Build history of the part. All positions in model axes, mm. A direction names the side the tool comes from. Coordinates: 2 decimals unless noted, no trailing zeros. Order: outer loops, then holes, each group sorted by start corner. A loop starts at its lowest first (then second) coordinate and runs counter-clockwise, first axis right, second up. Notation, with made-up numbers: (48, 81.5) -> (105, 81.5) arc R21 cw to (105, 93.5) -> close; hole circle Ø10 at (87, 52.5). An arc over 180 degrees is marked (long way). Write each question's results on one line, items separated by ' | '.
from build123d import *

# Parameters (mm, degrees)
F1_DEPTH = 40
F2_R     = 12.6
F3_T     = -4.129
F5_DEPTH = 14
F6_DEPTH = 20.001
F7_R     = 4.4681980282
F8_DEPTH = 12


with BuildPart() as f1:
    # F0 (on Top) → F1 (new body)
    with BuildSketch(Plane.XY):
        Polygon((-75.5, -10), (75.5, -10), (71.5217526524, 10), (-71.5217526524, 10), align=None)
    extrude(amount=F1_DEPTH)

    # F2
    f2_edges = [f1.edges().sort_by_distance(p)[0] for p in [
        (-71.521753, 10, 20),
        (0, 10, 40),
        (0, 10, 0),
        (71.521753, 10, 20),
        (-73.510876, 0, 40),
        (-73.510876, 0, 0),
        (73.510876, 0, 40),
        (73.510876, 0, 0),
    ]]
    fillet(f2_edges, radius=F2_R)

    # F3
    f3_openings = [f1.faces().sort_by_distance(p)[0] for p in [
        (0, -10, 20),
    ]]
    offset(amount=F3_T, openings=f3_openings)

    # F4 (on face) → F5 (join)
    with BuildSketch(Plane.XZ.offset(10)):
        with BuildLine():
            ThreePointArc((-71.2901081078, 22.15), (-69.7698285282, 21.5202795796), (-69.1401081078, 20))
            ThreePointArc((-69.1401081078, 20), (-69.7698285282, 18.4797204204), (-71.2901081078, 17.85))
            Line((-71.2901081078, 17.85), (-71.2901081078, 12.6))
            ThreePointArc((-71.2901081078, 12.6), (-63.8901081078, 20), (-71.2901081078, 27.4))
            Line((-71.2901081078, 27.4), (-71.2901081078, 22.15))
        make_face()
        with BuildLine():
            Line((71.2901081078, 22.15), (71.2901081078, 27.4))
            ThreePointArc((71.2901081078, 27.4), (63.8901081078, 20), (71.2901081078, 12.6))
            Line((71.2901081078, 12.6), (71.2901081078, 17.85))
            ThreePointArc((71.2901081078, 17.85), (69.1401081078, 20), (71.2901081078, 22.15))
        make_face()
    extrude(amount=-F5_DEPTH)

    # F4 (on face) → F6 (cut, through all)
    with BuildSketch(Plane.XZ.offset(10)):
        with BuildLine():
            ThreePointArc((-71.2901081078, 17.85), (-69.7698285282, 18.4797204204), (-69.1401081078, 20))
            ThreePointArc((-69.1401081078, 20), (-69.7698285282, 21.5202795796), (-71.2901081078, 22.15))
            Line((-71.2901081078, 22.15), (-71.2901081078, 17.85))
        make_face()
        with BuildLine():
            Line((-71.2901081078, 17.85), (-71.2901081078, 22.15))
            ThreePointArc((-71.2901081078, 22.15), (-73.4401081078, 20), (-71.2901081078, 17.85))
        make_face()
        with BuildLine():
            ThreePointArc((73.4401081078, 20), (72.8103876873, 21.5202795796), (71.2901081078, 22.15))
            Line((71.2901081078, 22.15), (71.2901081078, 17.85))
            ThreePointArc((71.2901081078, 17.85), (72.8103876873, 18.4797204204), (73.4401081078, 20))
        make_face()
        with BuildLine():
            Line((71.2901081078, 17.85), (71.2901081078, 22.15))
            ThreePointArc((71.2901081078, 22.15), (69.1401081078, 20), (71.2901081078, 17.85))
        make_face()
    extrude(amount=-F6_DEPTH, mode=Mode.SUBTRACT)

    # F7 (on face) → F8 (cut)
    with BuildSketch(Plane(origin=(0, 10, 0), x_dir=(-1, 0, 0), z_dir=(0, 1, 0))):
        with Locations((71.2666511536, 20.0136322528)):
            Circle(F7_R)
        with Locations((-71.2666511536, 20.0136322528)):
            Circle(F7_R)
    extrude(amount=-F8_DEPTH, mode=Mode.SUBTRACT)


solid = f1.part
Item 1: Tool access for faces 1 (the flat face through (-68.7, -2, 20.1)), 2 (the flat face through (65, 4, 20)), 3 (the flat face through (-1, -6, 40)), 4 (the cylindrical face through (-0.86, 3.46, 33.32)), 5 (the flat face through (74.533, -5.14, 19.896)): list every direction of +Z, -Z, +X, -X, +Y, -Y with a clear straight run to the whole face (end or side of a thin tool).
Answer:
face 1: +Y | face 2: none | face 3: +Z, +X, -X, +Y, -Y | face 4: -Y | face 5: +Z, -Z, +X, +Y
Item 2: Pin check, flat tips, straight feed: pin 1 (6 mm diameter, centred on y = 5.5, z = 16.5, fed in from -X); pin 2 (2 mm diameter, centred on x = 65, z = 22, fed in from +Y); pin 3 (0.8 mm diameter, centred on x = -65, z = 22, fed in from +Y). Stop position of each tip, or through.
Answer:
pin 1: stops at x = -72.66 | pin 2: stops at y = 9.68 | pin 3: stops at y = 9.53
Item 3: Slice it at B-B, the plane z = 8. List the corners of the cut face in (x, y).
Answer:
outline: (-74.61, -10) -> (-69.91, -10) -> (-68.16, -1.21) arc R7.11 cw to (-61.18, 4.51) -> (61.18, 4.51) arc R7.11 cw to (68.16, -1.21) -> (69.91, -10) -> (74.61, -10) -> (72.69, -0.31) arc R11.73 ccw to (61.18, 9.13) -> (-61.18, 9.13) arc R11.73 ccw to (-72.69, -0.31) -> close
Item 4: Slice it at A-A, the plane x = 7. List the corners of the cut face in (y, z), and give its area (3 significant figures).
Answer:
outline: (-10, 0) -> (-2.6, 0) arc R12.6 ccw to (10, 12.6) -> (10, 27.4) arc R12.6 ccw to (-2.6, 40) -> (-10, 40) -> (-10, 35.87) -> (-2.6, 35.87) arc R8.47 cw to (5.87, 27.4) -> (5.87, 12.6) arc R8.47 cw to (-2.6, 4.13) -> (-10, 4.13) -> close | area: 259 mm^2
Item 5: Pull direction X, two halves, no side cores. Call faces 6 (the cylindrical face through (-65.76, 9.14, 20.1)), 7 (the cylindrical face through (-63.89, -3.1, 19.84)), 8 (the cylindrical face through (-0.86, 6.41, 36.21)): released by +X, released by -X, zero draft, split by the parting line, or undercut.
Answer:
face 6: released by -X | face 7: undercut | face 8: zero draft
Item 6: Slice it at C-C, the plane y = -7.25. State how many separate pieces and enclosed holes the cut face has, and give its area (3 significant figures).
Answer:
separate pieces: 1 | enclosed holes: 3 | area: 1,560 mm^2
Item 7: Drill centre lines: line 1 (Z direction, x = 1, y = -2.25); line 2 (X direction, y = -6.25, z = 20); line 3 (X direction, y = -6.75, z = 20). Where is each one in solid material? Low to high. Write a range as from..to.
Answer:
line 1: z = 0..4.14, 35.86..40 | line 2: x = -74.75..-73.44, -69.14..-63.89, 63.89..69.14, 73.44..74.75 | line 3: x = -74.85..-73.44, -69.14..-63.89, 63.89..69.14, 73.44..74.85
